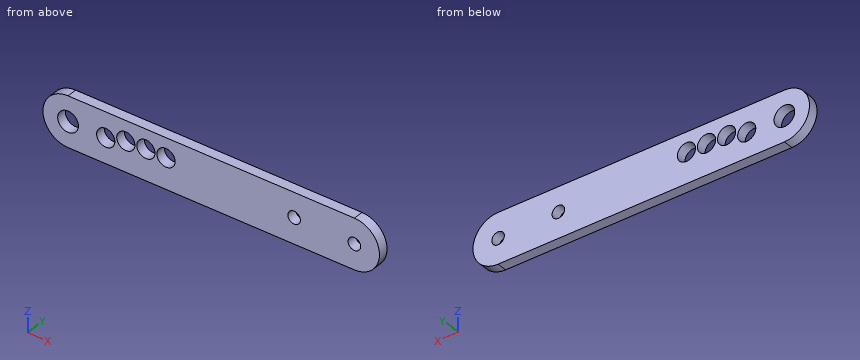
from build123d import *

# Parameters (mm, degrees)
F0_W      = 419.1
F0_H      = 88.9
F0_R      = 13.096875
F0_R_2    = 11.509375
F0_R_3    = 10.31875
F1_DEPTH  = 12.7
F2_R      = 11.509375
F3_DEPTH  = 12.701
F5_DEPTH  = 12.701
F7_DEPTH  = 12.7010001
F9_DEPTH  = 12.7
F10_R     = 13.096875
F10_R_2   = 11.509375
F10_R_3   = 7.9375
F11_DEPTH = 25.4010001


with BuildPart() as f1:
    # F0 (on Front) → F1 (new body)
    with BuildSketch(Plane.XZ):
        Rectangle(F0_W, F0_H)
        with Locations((-177.8, -12.7)):
            Circle(F0_R, mode=Mode.SUBTRACT)
        with Locations((-12.7, -18.7318846583)):
            Circle(F0_R_2, mode=Mode.SUBTRACT)
        with Locations((19.05, -19.1783625633)):
            Circle(F0_R_2, mode=Mode.SUBTRACT)
        with Locations((50.8, -18.7318846583)):
            Circle(F0_R_2, mode=Mode.SUBTRACT)
        with Locations((82.55, -19.05)):
            Circle(F0_R_2, mode=Mode.SUBTRACT)
        with Locations((133.35, -12.7)):
            Circle(F0_R_3, mode=Mode.SUBTRACT)
        with Locations((184.15, -12.7)):
            Circle(F0_R_3, mode=Mode.SUBTRACT)
    extrude(amount=-F1_DEPTH)

    # F2 (on face) → F3 (cut, through all)
    with BuildSketch(Plane.XZ):
        with Locations((-142.08252, 18.4232164174)):
            Circle(F2_R)
        with Locations((-104.306563735, 14.0248946846)):
            Circle(F2_R)
        with Locations((-71.5190842748, 1.6296281246)):
            Circle(F2_R)
        with Locations((-45.7596568011, -14.1053809535)):
            Circle(F2_R)
    extrude(amount=-F3_DEPTH, mode=Mode.SUBTRACT)

    # F4 (on face) → F5 (cut, through all)
    with BuildSketch(Plane.XZ):
        with BuildLine():
            ThreePointArc((-209.55, -12.7), (-207.0936907923, -0.4549120148), (-200.1048233219, 9.8955162937))
            Line((-200.1048233219, 9.8955162937), (-165.1, 44.45))
            Line((-165.1, 44.45), (-209.55, 44.45))
            Line((-209.55, 44.45), (-209.55, -12.7))
        make_face()
        with BuildLine():
            Line((-209.55, -44.45), (-177.8, -44.45))
            ThreePointArc((-177.8, -44.45), (-200.2506403027, -35.1506403027), (-209.55, -12.7))
            Line((-209.55, -12.7), (-209.55, -44.45))
        make_face()
        with BuildLine():
            ThreePointArc((-146.0861882684, -11.1845312756), (-146.0590483564, -11.9420496313), (-146.05, -12.7))
            ThreePointArc((-146.05, -12.7), (-155.3493596973, -35.1506403027), (-177.8, -44.45))
            Line((-177.8, -44.45), (-38.1, -44.45))
            add(Edge.make_bspline(
                [(-135.731991463, -1.5425124657), (-123.0853934374, -3.2529361125), (-97.8098704079, -7.8915227069), (-55.1757360667, -37.2664877617), (-44.6494842281, -43.1637651569), (-38.1, -44.45)],
                knots=[0, 0, 0, 0, 0.3555356426, 0.7550234425, 1, 1, 1, 1], degree=3))
            ThreePointArc((-135.731991463, -1.5425124657), (-142.8632378904, -4.2650367263), (-146.0861882684, -11.1845312756))
        make_face()
    extrude(amount=-F5_DEPTH, mode=Mode.SUBTRACT)

    # F6 (on face) → F7 (cut, through all)
    with BuildSketch(Plane.XZ):
        with BuildLine():
            Line((209.55, 44.45), (163.5125, 44.45))
            Line((163.5125, 44.45), (202.2463189928, 5.1236707474))
            ThreePointArc((202.2463189928, 5.1236707474), (207.6532604037, -3.0689694011), (209.55, -12.6999998198))
            Line((209.55, -12.6999998198), (209.55, 44.45))
        make_face()
        with BuildLine():
            Line((209.55, -44.45), (209.55, -12.6999998198))
            ThreePointArc((209.55, -12.6999998198), (206.8684506917, -24.0592252451), (199.39, -33.02))
            Line((199.39, -33.02), (184.15, -44.45))
            Line((184.15, -44.45), (209.55, -44.45))
        make_face()
    extrude(amount=-F7_DEPTH, mode=Mode.SUBTRACT)


with BuildPart() as f9:
    # F8 (on Front) → F9 (new body)
    with BuildSketch(Plane.XZ):
        with BuildLine():
            Line((180.975, 31.75), (-180.975, 31.75))
            ThreePointArc((-180.975, 31.75), (-212.725, 0), (-180.975, -31.75))
            Line((-180.975, -31.75), (180.975, -31.75))
            ThreePointArc((180.975, -31.75), (212.725, 0), (180.975, 31.75))
        make_face()
    extrude(amount=F9_DEPTH)


with BuildPart() as f11_tool:
    # F10 (on face) → F11 (new body, through all)
    with BuildSketch(Plane.XZ.offset(12.7)):
        with Locations((-180.975, 0)):
            Circle(F10_R)
        with Locations((-133.35, 0)):
            Circle(F10_R_2)
        with Locations((-107.95, 6.35)):
            Circle(F10_R_2)
        with Locations((-82.55, 7.0877922699)):
            Circle(F10_R_2)
        with Locations((-57.15, 7.0877922699)):
            Circle(F10_R_2)
        with Locations((104.7790011828, 0.7808740327)):
            Circle(F10_R_3)
        with Locations((180.975, 0)):
            Circle(F10_R_3)
    extrude(amount=-F11_DEPTH)


with BuildPart() as f1_1:
    add(f1.part)

    # F11: cut by f11_tool
    add(f11_tool.part, mode=Mode.SUBTRACT)


with BuildPart() as f9_1:
    add(f9.part)

    # F11: cut by f11_tool
    add(f11_tool.part, mode=Mode.SUBTRACT)


solid = f9_1.part
Can you work these out from the model? Positions are in its coordinate system, mm. Round coordinates to 2 decimals unless told otherwise and drop trailing zeros. Loops run counter-clockwise (first coordinate to the right, second up) from the corner with the lowest first, then second, coordinate; pieces in that order, holes last. Notation, with made-up numbers: (40.25, 45.5) - (59.25, 45.5) arc R16 cw to (59.25, 64.5) - close; hole circle Ø7 at (62.5, -34). An arc over 180 degrees is marked (long way). Answer in a Markdown table with one row per item. Add a question column.
Q1. I need wall thicknesses on L1, parallel to Z at x = -82.55, y = -4.5; L2, parallel to Z at x = -133.35, y = -7.5; L3, parallel to X at y = -6.75, z = 17. Which ranges of each line are inside material? Lowest first, please.
Q2. I want a section at A-A on x = -107.95. List the corners of the cut face in (y, z) for me.
Q3. I want a section at B-B on y = -6.5. Count the separate pieces of the cut face and the enclosed holes in it, and give its area (3 significant figures).
Q4. I want a section at C-C on z = -26.5. List the corners of the cut face in (x, y) for me, and give its area (3 significant figures).
Q5. For pin 1 Ø1.5 at (y, z) = (-4.5, 18.5) entering from +X; pin 2 Ø2 at (x, z) = (13, -10) entering from +Y; pin 3 Ø4 at (y, z) = (-8, 16.5) entering from -X, each with a flat end and sliding along its axis, tell me the tip position at first contact or that it passes through.
A:
| question | item | result |
|---|---|---|
| 1 | L1 | -31.75 to -4.42, 18.6 to 31.75 |
| 1 | L2 | -31.75 to -11.51, 11.51 to 31.75 |
| 1 | L3 | -207.79 to -112.31, -103.59 to -88.4, -76.7 to -63, -51.3 to 207.79 |
| 2 | outline | (-12.7, -31.75) - (0, -31.75) - (0, -5.16) - (-12.7, -5.16) - close; (-12.7, 17.86) - (0, 17.86) - (0, 31.75) - (-12.7, 31.75) - close |
| 3 | separate pieces | 1 |
| 3 | enclosed holes | 7 |
| 3 | area | 23,600 mm^2 |
| 4 | outline | (-198.46, -12.7) - (198.46, -12.7) - (198.46, 0) - (-198.46, 0) - close |
| 4 | area | 5,040 mm^2 |
| 5 | pin 1 | x = 207.3 |
| 5 | pin 2 | y = 0 |
| 5 | pin 3 | x = -209.22 |
